The drawing under review shows one solid part. Ordinate dimensions are in mm from its lowest x, y, z. Round coordinates to 2 decimals unless told otherwise and drop trailing zeros. Order: outer loops, then holes, each group sorted by start corner. A loop starts at its lowest first (then second) coordinate and runs counter-clockwise, first axis right, second up. Notation, with made-up numbers: M -11.5,-2.75 L 38.5,-2.75 A19 ccw 38.5,26.25 Z; hole C -29.5,23.5 d7. An arc over 180 degrees is marked long. Answer in a Markdown table with one row per item. Add a question column.
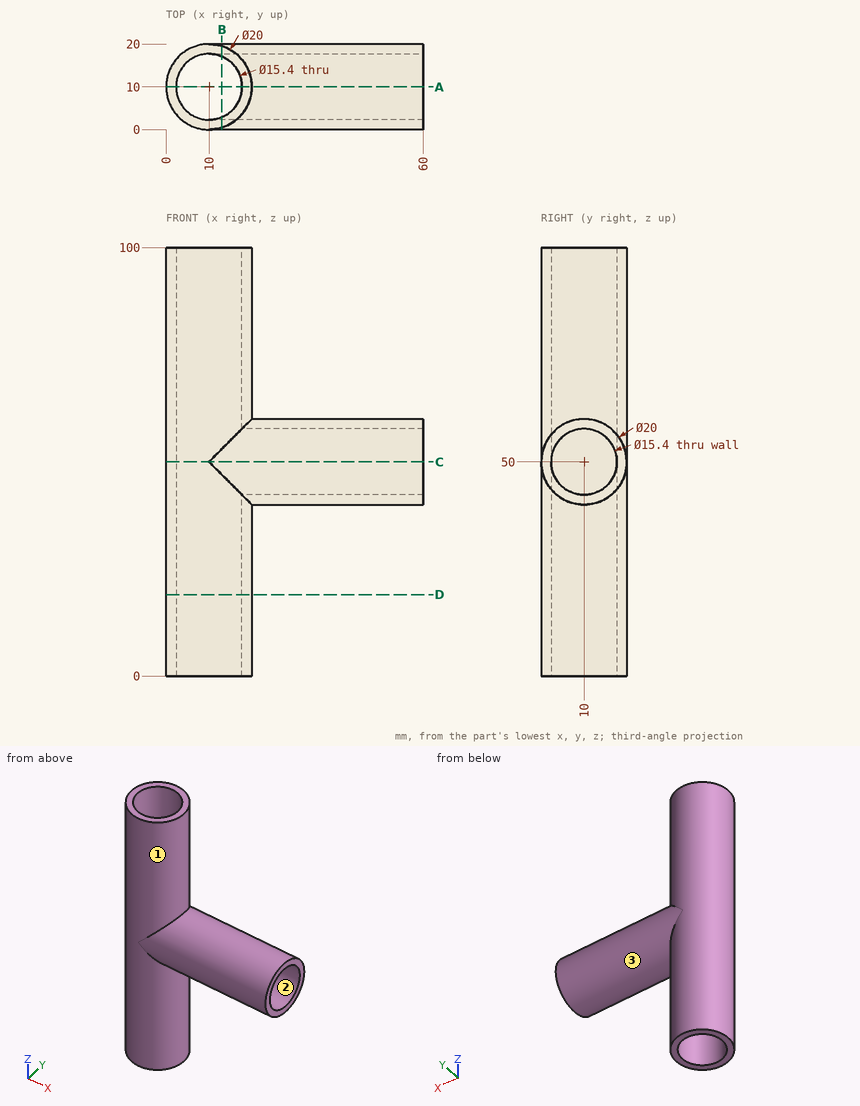
1. Consider section C-C on z = 50. Write out the cut boundary in (x, y).
2. To check wall thickness, follow probe 1 along Y at (x, z) = (10, 79); probe 2 along X at (y, z) = (12.75, 38); probe 3 along Y at (x, z) = (30, 45). State the ranges of each line that lie inside material, in increasing order. Write a range as [from, to].
3. Consider section D-D on z = 19. Write out the cut boundary in (x, y), plus the area to 3 significant figures.
4. Consider section A-A on y = 10. Write out the cut boundary in (x, z).
5. The part is to be moulded in two halves that separate along Z. For the marked faces 1, 2 and 3, say which applies: pulls with the +Z half, pulls with the -Z half, needs draft (parallel to the pull), parting line crosses it, or undercut.
6. Clearance check with flat-ended pins moving along their axes: pin 1 Ø5 at (x, y) = (40, 3) entering from -Z; pin 2 Ø1 at (y, z) = (9, 24.5) entering from +X; pin 3 Ø1 at (y, z) = (12, 70.5) entering from +X. State where each tip first meets the part, or that it passes through.
7. Consider section B-B on x = 13. Write out the cut boundary in (y, z).
Solved:
| question | item | result |
|---|---|---|
| 1 | outline | M 10,0 L 60,0 L 60,2.3 L 10,2.3 A7.7 cw 10,17.7 L 60,17.7 L 60,20 L 10,20 A10 ccw Z |
| 2 | probe 1 | y = [0, 2.3], [17.7, 20] |
| 2 | probe 2 | x = [0.39, 2.81], [17.19, 19.61] |
| 2 | probe 3 | y = [1.34, 4.14], [15.86, 18.66] |
| 3 | outline | C 10,10 d20; hole C 10,10 d15.4 |
| 3 | area | 128 mm^2 |
| 4 | outline | M 0,0 L 2.3,0 L 2.3,100 L 0,100 Z; M 17.7,0 L 20,0 L 20,40 L 60,40 L 60,42.3 L 17.7,42.3 Z; M 17.7,57.7 L 60,57.7 L 60,60 L 20,60 L 20,100 L 17.7,100 Z |
| 5 | face 1 | needs draft |
| 5 | face 2 | undercut |
| 5 | face 3 | parting line crosses it |
| 6 | pin 1 | stops at z = 41.07 |
| 6 | pin 2 | stops at x = 19.99 |
| 6 | pin 3 | stops at x = 19.89 |
| 7 | outline | M 0.46,0 L 2.91,0 L 2.91,47 A7.7 cw 2.91,53 L 2.91,100 L 0.46,100 L 0.46,53 A10 ccw 0.46,47 Z; M 17.09,0 L 19.54,0 L 19.54,47 A10 ccw 19.54,53 L 19.54,100 L 17.09,100 L 17.09,53 A7.7 cw 17.09,47 Z |
